Here's the drawing with two shaded views (mm, measured from the low corner). I have some questions. A direction names the side the tool comes from. Give positions to 0.01 mm unless a question says otherwise; leave off trailing zeros. Loops run counter-clockwise (first coordinate to the right, second up) from the corner with the lowest first, then second, coordinate; pieces in that order, holes last. Notation, with made-up numbers: (-26.5, 89) -> (-4.5, 89) arc R25 ccw to (-4.5, 103) -> close; hole circle Ø5 at (-31.75, 26.5). An arc over 180 degrees is marked (long way). Put each result on its own line as item: value.
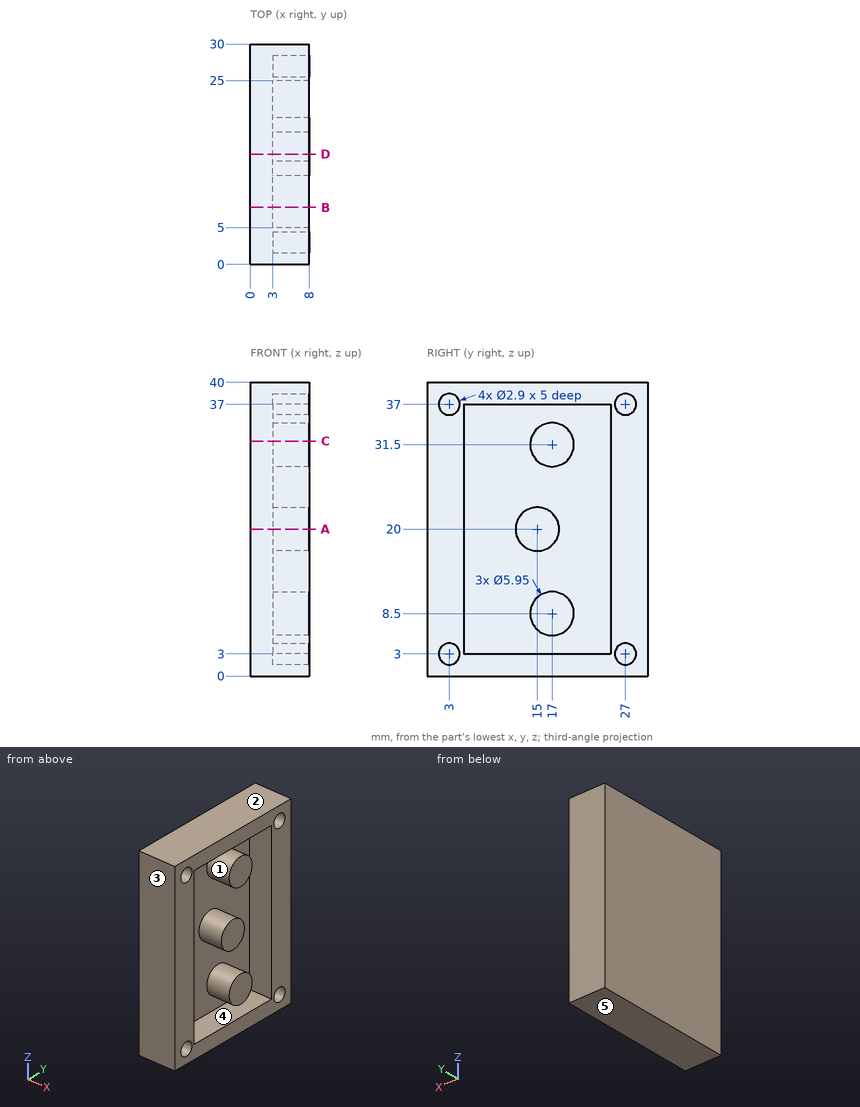
1. If we section it at C-C (z = 32): List the corners of the cut face in (x, y) for me.
Recorded:
outline: (0, 0) -> (8, 0) -> (8, 5) -> (3, 5) -> (3, 14.07) -> (8, 14.07) -> (8, 19.93) -> (3, 19.93) -> (3, 25) -> (8, 25) -> (8, 30) -> (0, 30) -> close
2. I need wall thicknesses on line 1 (Z direction, x = 7.5, y = 11); line 2 (Y direction, x = 6, z = 5); line 3 (X direction, y = 27.75, z = 38). Which ranges of each line are inside material? Lowest first, please.
Recorded:
line 1: z = 0 to 3, 37 to 40
line 2: y = 0 to 5, 25 to 30
line 3: x = 0 to 3
3. If we section it at B-B (y = 7.75): List the corners of the cut face in (x, z) for me.
Recorded:
outline: (0, 0) -> (8, 0) -> (8, 3) -> (3, 3) -> (3, 37) -> (8, 37) -> (8, 40) -> (0, 40) -> close
4. For the marked faces 4 and 5, which set-ups out of +Z, -Z, +X, -X, +Y, -Y let a thin tool reach every point of the face, with its end or its side?
Recorded:
face 4: +X
face 5: -Z, +X, -X, +Y, -Y
5. If we section it at A-A (z = 20): List the corners of the cut face in (x, y) for me (3 decimals).
Recorded:
outline: (0, 0) -> (8, 0) -> (8, 5) -> (3, 5) -> (3, 12.025) -> (8, 12.025) -> (8, 17.975) -> (3, 17.975) -> (3, 25) -> (8, 25) -> (8, 30) -> (0, 30) -> close
6. I'm going to push a flat-ended pin straight in: pin 1 (2.5 mm diameter, centred on y = 27, z = 37, fed in from +X). Where does the tip first touch, or does it pass through?
Recorded:
pin 1: stops at x = 3
7. Thinking about a two-plate mould opening in Y: for the marked faces 1, 2 and 3, which applies, pulls with the +Y half, pulls with the -Y half, needs draft (parallel to the pull), parting line crosses it, or undercut?
Recorded:
face 1: undercut
face 2: needs draft
face 3: pulls with the -Y half
8. If we section it at D-D (y = 15): List the corners of the cut face in (x, z) for me (3 decimals).
Recorded:
outline: (0, 0) -> (8, 0) -> (8, 3) -> (3, 3) -> (3, 6.298) -> (8, 6.298) -> (8, 10.702) -> (3, 10.702) -> (3, 17.025) -> (8, 17.025) -> (8, 22.975) -> (3, 22.975) -> (3, 29.298) -> (8, 29.298) -> (8, 33.702) -> (3, 33.702) -> (3, 37) -> (8, 37) -> (8, 40) -> (0, 40) -> close
